```python
from build123d import *

# Parameters (mm, degrees)
F1_DEPTH = 17.5
F2_R     = 4
F3_DEPTH = 25
F4_R     = 4.4
F5_DEPTH = 25
F6_R     = 2


# Not quite as in the source:
# - a feature names something its author has since deleted; it is built from what else it names


with BuildPart() as f1:
    # F0 (on Front) → F1 (new body, symmetric)
    with BuildSketch(Plane.XZ):
        Polygon((95, -38), (95, 5), (-95, 5), (-95, -38), (-115, -38), (-115, -40), (-93, -40), (-93, 3), (93, 3), (93, -40), (115, -40), (115, -38), align=None)
    extrude(amount=F1_DEPTH, both=True)

    # F2 (on face) → F3 (cut)
    with BuildSketch(Plane.XY.offset(-38)):
        with Locations((-105, 0)):
            Circle(F2_R)
        with Locations((105, 0)):
            Circle(F2_R)
    extrude(amount=-F3_DEPTH, mode=Mode.SUBTRACT)

    # F4 (on face) → F5 (cut)
    with BuildSketch(Plane.XY.offset(5)):
        with Locations((-32.5, 0)):
            Circle(F4_R)
        with Locations((32.5, 0)):
            Circle(F4_R)
    extrude(amount=-F5_DEPTH, mode=Mode.SUBTRACT)

    # F6
    f6_edges = [f1.edges().sort_by_distance(p)[0] for p in [
        (95, 0, 5),
        (-95, 0, 5),
        (-93, 0, -40),
        (93, 0, -40),
    ]]
    fillet(f6_edges, radius=F6_R)


solid = f1.part
```
Model file for the job. Use its own axes, mm. A direction names the side the tool comes from. Give positions to 0.01 mm unless a question says otherwise; leave off trailing zeros. Write each loop counter-clockwise with the first axis right and the second up, starting at its lowest first coordinate (ties: lowest second). Pieces come first, ordered by that corner, then holes. Notation, with made-up numbers: (-15, -33) - (-8, -33) arc R22 cw to (-8, 3) - close; hole circle Ø4 at (7, -12). An arc over 180 degrees is marked (long way). One line per question, with ' | ' between items. Start each with the question number.
(1) Two-plate mould, pull along X, no slides. Class faces 1 (the face through (1, 0, 5)), 2 (the face through (95, 0, -18)), 3 (the face through (93, 0, -17)): +X half, -X half, draft (parallel to the pull), parting line (faces both ways), or undercut.
(2) Slice it at A-A on x = -32.5. Write the cut outline in (y, z).
(3) Slice it at C-C on y = 0. Give the number of separate pieces and of enclosed holes in the cut face, plus the area to 3 significant figures.
(4) Pin check, flat tips, straight feed: P1, Ø10.5, axis at y = -8.5, z = -20.5, coming from the +X side; P2, Ø16, axis at x = -103.5, y = 8.5, coming from the +Z side; P3, Ø14, axis at x = 32.5, y = 0, coming from the -Z side; P4, Ø5, axis at x = -105, y = 0, coming from the -Z side. Stop position of each tip, or through.
(5) Slice it at D-D on y = -9.5. Write the cut outline in (x, z), plus the area to 3 significant figures.
(6) Slice it at B-B on z = -36. Write the cut outline in (x, y), plus the area to 3 significant figures.
(7) 3-axis set-ups, long thin cutter, end or side, ignore diameter. For faces 4 (the face through (-1, 0, 3)), 5 (the face through (107, -4, -38)), 6 (the face through (-95, 0, -17)): which of +Z, -Z, +X, -X, +Y, -Y reach the whole face in a straight line?
(8) Wall check: line 1 along X through (y, z) = (13.5, -18.5); line 2 along Y through (x, z) = (105, -38.95); line 3 along Z through (x, y) = (83, 2). Give the ranges that are in metal, low to high. Write a range as from..to.
Results below:
1) face 1: draft | face 2: +X half | face 3: undercut
2) outline: (-17.5, 3) - (-4.4, 3) - (-4.4, 5) - (-17.5, 5) - close; (4.4, 3) - (17.5, 3) - (17.5, 5) - (4.4, 5) - close
3) separate pieces: 5 | enclosed holes: 0 | area: 561 mm^2
4) P1: x = 95 | P2: z = -38 | P3: z = 3 | P4: through
5) outline: (-115, -40) - (-95, -40) arc R2 ccw to (-93, -38) - (-93, 3) - (93, 3) - (93, -38) arc R2 ccw to (95, -40) - (115, -40) - (115, -38) - (95, -38) - (95, 3) arc R2 ccw to (93, 5) - (-93, 5) arc R2 ccw to (-95, 3) - (-95, -38) - (-115, -38) - close | area: 629 mm^2
6) outline: (-95, -17.5) - (-93, -17.5) - (-93, 17.5) - (-95, 17.5) - close; (93, -17.5) - (95, -17.5) - (95, 17.5) - (93, 17.5) - close | area: 140 mm^2
7) face 4: -Z, +Y, -Y | face 5: +Z, +X, +Y, -Y | face 6: +Z, -X, +Y, -Y
8) line 1: -95..-93, 93..95 | line 2: -17.5..-4, 4..17.5 | line 3: 3..5
